from build123d import *

# Parameters (mm, degrees)
SKETCH_2_R               = 10
EXTRUDE_1_DEPTH          = 6
SKETCH_3_R               = 15
EXTRUDE_2_DEPTH          = 2
EXTRUDE_START            = 2
SKETCH_4_R               = 15
EXTRUDE_3_DEPTH          = 2
CUT_EXTRUDE_1_DEPTH      = 24.452078799
CUT_EXTRUDE_1_DEPTH_BACK = 24.452078799
SKETCH_5_R               = 7.5
CUT_EXTRUDE_2_DEPTH      = 24.452078799
CUT_EXTRUDE_2_DEPTH_BACK = 24.452078799
SKETCH_6_R               = 1.351786052


with BuildPart() as part:
    # 스케치2 → 보스-돌출1 (new body)
    with BuildSketch(Plane.XY):
        Circle(SKETCH_2_R)
    extrude(amount=EXTRUDE_1_DEPTH)

    # 스케치3 → 보스-돌출2 (add)
    with BuildSketch(Plane(origin=(0, 0, 0), x_dir=(-1, 0, 0), z_dir=(0, 0, -1))):
        Circle(SKETCH_3_R)
    extrude(amount=EXTRUDE_2_DEPTH)

    # 스케치4 → 보스-돌출3 (add)
    with BuildSketch(Plane.XY.offset(6).offset(EXTRUDE_START)):
        with Locations(Location((0, 0, 0), (0, 0, 180))):
            Circle(SKETCH_4_R)
    extrude(amount=-EXTRUDE_3_DEPTH)

    # 스케치5 → 컷-돌출1 (cut, two sides: drawn at the far end of the back side and taken through both)
    with BuildSketch(Plane.XY.offset(8).offset(-CUT_EXTRUDE_1_DEPTH_BACK)):
        Circle(SKETCH_5_R)
    extrude(amount=CUT_EXTRUDE_1_DEPTH + CUT_EXTRUDE_1_DEPTH_BACK, mode=Mode.SUBTRACT)

    # 스케치6 → 컷-돌출2 (cut, two sides: drawn at the far end of the back side and taken through both)
    with BuildSketch(Plane.XY.offset(8).offset(-CUT_EXTRUDE_2_DEPTH_BACK)):
        with Locations((13.094626163, 0)):
            Circle(SKETCH_6_R)
    extrude(amount=CUT_EXTRUDE_2_DEPTH + CUT_EXTRUDE_2_DEPTH_BACK, mode=Mode.SUBTRACT)


solid = part.part
Geometry check sheet. Reference: the model listing, model coordinates, mm. A direction names the side the tool comes from. Coordinates: 2 decimals unless noted, no trailing zeros. Order: outer loops, then holes, each group sorted by start corner. A loop starts at its lowest first (then second) coordinate and runs counter-clockwise, first axis right, second up. Notation, with made-up numbers: (-26.5, 28.25) - (-17.5, 28.25) arc R29 cw to (-17.5, 53.25) - close; hole circle Ø1 at (-29.75, 16.25). An arc over 180 degrees is marked (long way). Answer in a Markdown table with one row per item. Add a question column.
1) Cross-section at B-B, the plane y = 0. Record the cut outline in (x, z).
2) Cross-section at D-D, the plane x = 8.25. Record the cut outline in (y, z), then the cut area to 3 significant figures.
3) Material ranges on line 1 along Y through (x, z) = (0, 3.25); line 2 along Y through (x, z) = (0.25, 7.5); line 3 along Z through (x, y) = (5.25, 9), recorded low to high. Write a range as [from, to].
4) Release check for a two-part mould opening along Z. For faces 1 (the cylindrical face through (14.384, 0.406, 6.986)), 2 (the flat face through (4, 7, -2)), 3 (the flat face through (4, -7, 8)), 4 (the cylindrical face through (-2.17, -9.76, 2.96)) record: +Z half, -Z half, draft (parallel to the pull), parting line (faces both ways), or undercut.
5) Cross-section at A-A, the plane x = 0. Record the cut outline in (y, z).
6) Set-up check for faces 5 (the flat face through (-10, 3, 6)), 6 (the cylindrical face through (-7.493, 0.33, 2.93)): record each of +Z, -Z, +X, -X, +Y, -Y from which the full face is reachable in a straight line by a thin tool's end or side.
7) Gauge pin test, flat ends, axial feed: P1, Ø3, axis at y = 11, z = 7, coming from the -X side; P2, Ø1.5, axis at x = -1, z = 3.5, coming from the +Y side; P3, Ø2, axis at y = 8, z = 0, coming from the -X side; P4, Ø12, axis at x = 0, y = 0, coming from the -Z side. Record the tip position at first contact, or that the pin passes through.
8) Cross-section at C-C, the plane y = -3.25. Record the cut outline in (x, z).
Check result:
| question | item | result |
|---|---|---|
| 1 | outline | (-15, -2) - (-7.5, -2) - (-7.5, 8) - (-15, 8) - (-15, 6) - (-10, 6) - (-10, 0) - (-15, 0) - close; (7.5, -2) - (11.74, -2) - (11.74, 0) - (10, 0) - (10, 6) - (11.74, 6) - (11.74, 8) - (7.5, 8) - close; (14.45, -2) - (15, -2) - (15, 0) - (14.45, 0) - close; (14.45, 6) - (15, 6) - (15, 8) - (14.45, 8) - close |
| 2 | outline | (-12.53, -2) - (12.53, -2) - (12.53, 0) - (5.65, 0) - (5.65, 6) - (12.53, 6) - (12.53, 8) - (-12.53, 8) - (-12.53, 6) - (-5.65, 6) - (-5.65, 0) - (-12.53, 0) - close |
| 2 | area | 168 mm² |
| 3 | line 1 | y = [-10, -7.5], [7.5, 10] |
| 3 | line 2 | y = [-15, -7.5], [7.5, 15] |
| 3 | line 3 | z = [-2, 0], [6, 8] |
| 4 | face 1 | draft |
| 4 | face 2 | -Z half |
| 4 | face 3 | +Z half |
| 4 | face 4 | undercut |
| 5 | outline | (-15, -2) - (-7.5, -2) - (-7.5, 8) - (-15, 8) - (-15, 6) - (-10, 6) - (-10, 0) - (-15, 0) - close; (7.5, -2) - (15, -2) - (15, 0) - (10, 0) - (10, 6) - (15, 6) - (15, 8) - (7.5, 8) - close |
| 6 | face 5 | none |
| 6 | face 6 | +Z, -Z |
| 7 | P1 | stops at x = -11.61 |
| 7 | P2 | stops at y = 10 |
| 7 | P3 | stops at x = -13.27 |
| 7 | P4 | passes through |
| 8 | outline | (-14.64, -2) - (-6.76, -2) - (-6.76, 8) - (-14.64, 8) - (-14.64, 6) - (-9.46, 6) - (-9.46, 0) - (-14.64, 0) - close; (6.76, -2) - (14.64, -2) - (14.64, 0) - (9.46, 0) - (9.46, 6) - (14.64, 6) - (14.64, 8) - (6.76, 8) - close |
